Can you work these out from the model? Positions are in its coordinate system, mm. A direction names the side the tool comes from. Give positions to 0.01 mm unless a question says otherwise; leave off trailing zeros. Write each loop counter-clockwise with the first axis right and the second up, starting at its lowest first coordinate (ties: lowest second). Pieces come first, ordered by that corner, then holes.
1. Suppose I cut it at A-A (x = 0). Please give me the cut outline in (y, z), and give its area (3 significant figures).
2. I'm going to push flat-ended pins straight in: pin 1 (2 mm diameter, centred on y = 4, z = -24, fed in from -X); pin 2 (1.5 mm diameter, centred on x = -13.5, z = -3.5, fed in from -Y). Where does each tip first touch, or does it pass through?
3. If I drill on probe 1 along X at (y, z) = (1.05, 0); probe 2 along X at (y, z) = (4.35, 0); probe 3 along Z at (x, y) = (24, 0.5), over which ranges is the centre line in solid material (lowest first)?
4. On a 3-axis mill with a long thin cutter (end or side, diameter ignored), from which of +Z, -Z, +X, -X, +Y, -Y can I reach the whole of each face in a straight line? I mean faces 1 (the flat face through (-13, 0, 13)), 2 (the cylindrical face through (5.407, 0.197, -17.169)), 3 (the flat face through (13, 1.52, -3)). Say none if no direction works.
5. Thinking about a two-plate mould opening in X: for faces 4 (the cylindrical face through (-10.648, 3.791, -13.887)), 5 (the cylindrical face through (-7.91, 0.968, -10.316)), 6 (the flat face through (25, 5, -9)), 7 (the cylindrical face through (-15.821, 5.493, -20.633)), which applies, pulls with the +X half, pulls with the -X half, needs draft (parallel to the pull), parting line crosses it, or undercut?
6. Suppose I cut it at C-C (y = 4.05). Please give me the cut outline in (x, z).
7. Suppose I cut it at D-D (x = 19.5). Please give me the cut outline in (y, z), and give its area (3 significant figures).
8. Suppose I cut it at B-B (z = 0). Please give me the cut outline in (x, y).
```python
from build123d import *

# Parameters (mm, degrees)
SKETCH_1_R          = 30
EXTRUDE_1_DEPTH     = 5
SKETCH_2_R          = 26
EXTRUDE_2_DEPTH     = 1
SKETCH_3_R          = 18
CUT_EXTRUDE_1_DEPTH = 0.4
SKETCH_4_R          = 17.5
CUT_EXTRUDE_2_DEPTH = 4.48
SKETCH_5_R          = 13
CUT_EXTRUDE_3_DEPTH = 43.662283108


with BuildPart() as part:
    # 草图1 → 凸台-拉伸1 (new body)
    with BuildSketch(Plane(origin=(0, 0, 0), x_dir=(1, 0, 0), z_dir=(0, 1, 0))):
        with Locations(Location((0, 0, 0), (0, 0, 270))):
            Circle(SKETCH_1_R)
    extrude(amount=EXTRUDE_1_DEPTH)

    # 草图2 → 凸台-拉伸2 (add)
    with BuildSketch(Plane(origin=(0, 5, 0), x_dir=(1, 0, 0), z_dir=(0, 1, 0))):
        with Locations(Location((0, 0, 0), (0, 0, 270))):
            Circle(SKETCH_2_R)
    extrude(amount=EXTRUDE_2_DEPTH)

    # 草图3 → 切除-拉伸1 (cut)
    with BuildSketch(Plane.XZ):
        with Locations(Location((0, 0, 0), (0, 0, 270))):
            Circle(SKETCH_3_R)
    extrude(amount=-CUT_EXTRUDE_1_DEPTH, mode=Mode.SUBTRACT)

    # 草图4 → 切除-拉伸2 (cut)
    with BuildSketch(Plane(origin=(0, 6, 0), x_dir=(1, 0, 0), z_dir=(0, 1, 0))):
        with Locations(Location((0, 0, 0), (0, 0, 270))):
            Circle(SKETCH_4_R)
    extrude(amount=-CUT_EXTRUDE_2_DEPTH, mode=Mode.SUBTRACT)

    # 草图5 → 切除-拉伸3 (cut, through all)
    with BuildSketch(Plane(origin=(0, 1.52, 0), x_dir=(1, 0, 0), z_dir=(0, 1, 0))):
        with Locations(Location((0, 0, 0), (0, 0, 270))):
            Circle(SKETCH_5_R)
    extrude(amount=-CUT_EXTRUDE_3_DEPTH, mode=Mode.SUBTRACT)


solid = part.part
```
Checks:
1. outline: (0, -30) - (5, -30) - (5, -26) - (6, -26) - (6, -17.5) - (1.52, -17.5) - (1.52, -13) - (0.4, -13) - (0.4, -18) - (0, -18) - close; (0, 18) - (0.4, 18) - (0.4, 13) - (1.52, 13) - (1.52, 17.5) - (6, 17.5) - (6, 26) - (5, 26) - (5, 30) - (0, 30) - close
1. area: 152 mm2
2. pin 1: stops at x = -19.26
2. pin 2: stops at y = 0.4
3. probe 1: x = -30 to -13, 13 to 30
3. probe 2: x = -30 to -17.5, 17.5 to 30
3. probe 3: z = -18 to 18
4. face 1: +Z, -Z, +X, -X, -Y
4. face 2: -Y
4. face 3: +Y
5. face 4: undercut
5. face 5: undercut
5. face 6: needs draft
5. face 7: parting line crosses it
6. outline: circle Ø60 at (0, 0); hole circle Ø35 at (0, 0)
7. outline: (0, -22.8) - (5, -22.8) - (5, -17.2) - (6, -17.2) - (6, 17.2) - (5, 17.2) - (5, 22.8) - (0, 22.8) - close
7. area: 262 mm2
8. outline: (-30, 0) - (-18, 0) - (-18, 0.4) - (-13, 0.4) - (-13, 1.52) - (-17.5, 1.52) - (-17.5, 6) - (-26, 6) - (-26, 5) - (-30, 5) - close; (13, 0.4) - (18, 0.4) - (18, 0) - (30, 0) - (30, 5) - (26, 5) - (26, 6) - (17.5, 6) - (17.5, 1.52) - (13, 1.52) - close
